```python
from build123d import *

# Parameters (mm, degrees)
SKETCH_1_R      = 260
EXTRUDE_3_DEPTH = 16


with BuildPart() as part:
    # Эскиз1 → Бобышка-Вытянуть3 (new body)
    with BuildSketch(Plane(origin=(0, 0, 0), x_dir=(1, 0, 0), z_dir=(0, 1, 0))):
        with BuildLine():
            Line((-564.131109826, 487.398330281), (-548.396606244, 484.495676837))
            Line((-548.396606244, 484.495676837), (-544.787643902, 504.058890969))
            ThreePointArc((-544.787643902, 504.058890969), (-360.125373537, 380.954998191), (-310.604335978, 164.61639934))
            Line((-310.604335978, 164.61639934), (-330.255153903, 167.66400738))
            Line((-330.255153903, 167.66400738), (-333.157807348, 151.929503798))
            Line((-333.157807348, 151.929503798), (-313.713053206, 147.764879413))
            ThreePointArc((-313.713053206, 147.764879413), (-436.861002003, -36.453770733), (-652.865766443, -85.889285226))
            Line((-652.865766443, -85.889285226), (-649.829869088, -66.239005386))
            Line((-649.829869088, -66.239005386), (-665.565211025, -63.340900125))
            Line((-665.565211025, -63.340900125), (-669.719078569, -82.790306674))
            ThreePointArc((-669.719078569, -82.790306674), (-854.107254512, 40.393898968), (-903.516250652, 256.569982398))
            Line((-903.516250652, 256.569982398), (-883.865432727, 253.522374358))
            Line((-883.865432727, 253.522374358), (-880.962779283, 269.256877941))
            Line((-880.962779283, 269.256877941), (-900.525993415, 272.865840282))
            ThreePointArc((-900.525993415, 272.865840282), (-777.422100637, 457.528110648), (-561.083501786, 507.049148206))
            Line((-561.083501786, 507.049148206), (-564.131109826, 487.398330281))
        make_face()
        with Locations((-607.060293315, 210.593190869)):
            Circle(SKETCH_1_R, mode=Mode.SUBTRACT)
    extrude(amount=EXTRUDE_3_DEPTH)


solid = part.part
```
Read the model definition and answer for the solid it produces. Units are mm, in the model's axes. A direction names the side the tool comes from. Give positions to 0.01 mm unless a question says otherwise; leave off trailing zeros. Order: outer loops, then holes, each group sorted by start corner. A loop starts at its lowest first (then second) coordinate and runs counter-clockwise, first axis right, second up. Notation, with made-up numbers: (48, 30) -> (73, 30) arc R18 cw to (73, 59) -> close; hole circle Ø5 at (49, 29.25). An arc over 180 degrees is marked (long way). One line per item, written item: value. Start each with the question number.
(1) Flat-ended cylindrical pins translate along their axes: P1, Ø4, axis at x = -828.5, z = -410.5, coming from the -Y side; P2, Ø4, axis at y = 9.5, z = -209, coming from the +X side; P3, Ø1, axis at y = 8.5, z = -15, coming from the +X side; P4, Ø5, axis at x = -668.5, y = 13, coming from the -Z side. Find the tip coordinate at first contact, or state that the pin passes through.
(2) The part is cut by section C-C (y = 5.5). Determine the outline of the cut face in (x, z), and give its area (3 significant figures).
(3) A tool of negligible diameter and unlimited length cuts with its end or side. For faces 1 (the flat face through (-893.828, 7.888, -255.068)), 2 (the flat face through (-361, 0, -301)), 3 (the flat face through (-890.607, 7.888, -271.036)), 4 (the flat face through (-323.572, 7.888, -149.876)), 5 (the flat face through (-546.617, 7.888, -494.14)), from which of +Z, -Z, +X, -X, +Y, -Y can it reach the whole face along a straight path? Write none if from no direction.
(4) Straight lines are drawn through the part: L1, parallel to Z at x = -393, y = 10.5; L2, parallel to X at y = 10, z = -281; L3, parallel to Z at x = -595.5, y = 8. For each, find the intervals that lie inside material, in ascending order.
(5) For a pull along Z with two mould halves and no side action, classify faces 6 (the flat face through (-667.613, 7.888, 72.929)), 7 (the flat face through (-651.37, 7.89, 76.2)), 8 (the cylindrical face through (-780.03, 7.89, -455.71)) as released by +Z, released by -Z, zero draft, split by the parting line, or undercut.
(6) The part is cut by section A-A (z = -197.5). Determine the outline of the cut face in (x, y).
(7) The part is cut by section B-B (x = -479). Determine the outline of the cut face in (y, z), and give its area (3 significant figures).
Taken from the geometry:
1. P1: y = 0
1. P2: x = -307.06
1. P3: x = -379.16
1. P4: z = -504.75
2. outline: (-903.52, -256.57) -> (-883.87, -253.52) -> (-880.96, -269.26) -> (-900.53, -272.87) arc R300 ccw to (-561.08, -507.05) -> (-564.13, -487.4) -> (-548.4, -484.5) -> (-544.79, -504.06) arc R300 ccw to (-310.6, -164.62) -> (-330.26, -167.66) -> (-333.16, -151.93) -> (-313.71, -147.76) arc R300 ccw to (-652.87, 85.89) -> (-649.83, 66.24) -> (-665.57, 63.34) -> (-669.72, 82.79) arc R300 ccw to start; hole circle Ø520 at (-607.06, -210.59)
2. area: 69,100 mm^2
3. face 1: +Y, -Y
3. face 2: +Z, -Z, +X, -X, -Y
3. face 3: -X, +Y, -Y
3. face 4: +X, +Y, -Y
3. face 5: -Z, +Y, -Y
4. L1: -420.78 to -358.17, -63.02 to -0.41
4. L2: -898.68 to -857.35, -356.77 to -315.44
4. L3: -510.37 to -470.34, 49.15 to 89.18
5. face 6: released by +Z
5. face 7: undercut
5. face 8: released by -Z
6. outline: (-906.77, 0) -> (-866.73, 0) -> (-866.73, 16) -> (-906.77, 16) -> close; (-347.39, 0) -> (-307.35, 0) -> (-307.35, 16) -> (-347.39, 16) -> close
7. outline: (0, -481.89) -> (16, -481.89) -> (16, -436.87) -> (0, -436.87) -> close; (0, 15.68) -> (16, 15.68) -> (16, 60.7) -> (0, 60.7) -> close
7. area: 1,440 mm^2
